from build123d import *

# Parameters (mm, degrees)
F0_R     = 3.175
F1_DEPTH = 19.05
F2_R     = 3.175
F3_DEPTH = 9.525
F4_W     = 15.875
F4_H     = 31.190733
F5_DEPTH = 9.525
F6_R     = 3.175
F7_DEPTH = 20.32
F8_R     = 3.175
F9_DEPTH = 20.32


with BuildPart() as f1:
    # F0 (on Top) → F1 (new body)
    with BuildSketch(Plane.XY):
        with BuildLine():
            ThreePointArc((100.157061, 0.559267), (119.207061, 19.609267), (100.157061, 38.659267))
            Line((100.157061, 38.659267), (-97.640359, 38.659267))
            ThreePointArc((-97.640359, 38.659267), (-116.690359, 19.609267), (-97.640359, 0.559267))
            Line((-97.640359, 0.559267), (100.157061, 0.559267))
        make_face()
        with Locations((-97.640359, 19.609267)):
            Circle(F0_R, mode=Mode.SUBTRACT)
        with Locations((100.157061, 19.609267)):
            Circle(F0_R, mode=Mode.SUBTRACT)
    extrude(amount=F1_DEPTH)

    # F2 (on face) → F3 (cut)
    with BuildSketch(Plane.XY.offset(19.05)):
        with Locations((-97.640359, 19.609267)):
            Circle(F2_R)
        with Locations((100.157061, 19.609267)):
            Circle(F2_R)
        with BuildLine():
            ThreePointArc((100.149441, -5.790733), (125.549441, 19.609267), (100.149441, 45.009267))
            Line((100.149441, 45.009267), (36.649441, 45.009267))
            Line((36.649441, 45.009267), (36.649441, -5.790733))
            Line((36.649441, -5.790733), (100.149441, -5.790733))
        make_face()
        with Locations((100.157061, 19.609267)):
            Circle(F2_R, mode=Mode.SUBTRACT)
        with BuildLine():
            Line((-34.140359, -5.790733), (-34.140359, 45.009267))
            Line((-34.140359, 45.009267), (-97.640359, 45.009267))
            ThreePointArc((-97.640359, 45.009267), (-123.040359, 19.609267), (-97.640359, -5.790733))
            Line((-97.640359, -5.790733), (-34.140359, -5.790733))
        make_face()
        with Locations((-97.640359, 19.609267)):
            Circle(F2_R, mode=Mode.SUBTRACT)
    extrude(amount=-F3_DEPTH, mode=Mode.SUBTRACT)

    # F4 (on face) → F5 (cut)
    with BuildSketch(Plane(origin=(0, 0, 0), x_dir=(1, 0, 0), z_dir=(0, 0, -1))):
        Polygon((-15.875, 0), (-15.875, -19.609267), (0, -19.609267), (15.875, -19.609267), (15.875, 0), align=None)
        with Locations((-7.9375, -35.204633)):
            Rectangle(F4_W, F4_H)
        with Locations((7.9375, -35.204633)):
            Rectangle(F4_W, F4_H)
    extrude(amount=-F5_DEPTH, mode=Mode.SUBTRACT)

    # F6 (on face) → F7 (join)
    with BuildSketch(Plane(origin=(0, 0, 0), x_dir=(1, 0, 0), z_dir=(0, 0, -1))):
        with Locations((-97.640359, -19.609267)):
            Circle(F6_R)
    extrude(amount=-F7_DEPTH)

    # F8 (on face) → F9 (join)
    with BuildSketch(Plane(origin=(0, 0, 0), x_dir=(1, 0, 0), z_dir=(0, 0, -1))):
        with Locations((100.157061, -19.609267)):
            Circle(F8_R)
    extrude(amount=-F9_DEPTH)


solid = f1.part
Work out the finished part from the listing and answer in its coordinate system (mm). A direction names the side the tool comes from. Round coordinates to 2 decimals unless told otherwise and drop trailing zeros. Write each loop counter-clockwise with the first axis right and the second up, starting at its lowest first coordinate (ties: lowest second). Pieces come first, ordered by that corner, then holes.
1) A cutting plane is placed at C-C (x = -59.5). Give the vertices of the cut face in (y, z) (3 decimals).
2) A tool of negligible diameter and unlimited length cuts with its end or side. For faces 4 (the flat face through (15.875, 20, 5)), 5 (the cylindrical face through (-116.686, 20.028, 4.696)), 6 (the cylindrical face through (-94.71, 20.83, 14.85)), from which of +Z, -Z, +X, -X, +Y, -Y can it reach the whole face along a straight path? Write none if from no direction.
3) A cutting plane is placed at D-D (y = 33). Give the vertices of the cut face in (x, z) (3 decimals), plus the area to 3 significant figures.
4) Straight lines are drawn through the part: line 1 (X direction, y = 21, z = 17.5); line 2 (Z direction, x = 53.5, y = 6) (3 decimals); line 3 (Z direction, x = -17, y = 10.5). For each, find the intervals that lie inside material, in ascending order.
5) The mould has two halves that part along X. Classify faces 1 (the flat face through (-15.875, 19, 5)), 2 (the flat face through (100, 20, 20.32)), 3 (the cylindrical face through (119.202, 19.19, 4.696)): pulls with the +X half, pulls with the -X half, needs draft (parallel to the pull), parting line crosses it, or undercut.
6) A cutting plane is placed at B-B (y = 6.5). Give the vertices of the cut face in (x, z) (3 decimals).
7) Given pin 1 Ø10.5 at (y, z) = (24.5, 15.5) entering from +X; pin 2 Ø1 at (y, z) = (17, 11) entering from +X; pin 3 Ø3 at (y, z) = (24, 14) entering from -X, each flat-ended and moving along its own axis, determine where each tip first touches the part or whether it passes through.
8) A cutting plane is placed at A-A (z = 4.75). Give the vertices of the cut face in (x, y) (3 decimals).
Completed:
1. outline: (0.559, 0) - (38.659, 0) - (38.659, 9.525) - (0.559, 9.525) - close
2. face 4: -Z, +Y, -Y
2. face 5: +Z, -Z, -X
2. face 6: +Z
3. outline: (-111.19, 0) - (-15.875, 0) - (-15.875, 9.525) - (15.875, 9.525) - (15.875, 0) - (113.707, 0) - (113.707, 9.525) - (36.649, 9.525) - (36.649, 19.05) - (-34.14, 19.05) - (-34.14, 9.525) - (-111.19, 9.525) - close
3. area: 2,510 mm2
4. line 1: x = -100.49 to -94.79, -34.14 to 36.65, 97.3 to 103.01
4. line 2: z = 0 to 9.525
4. line 3: z = 0 to 19.05
5. face 1: undercut
5. face 2: needs draft
5. face 3: pulls with the +X half
6. outline: (-111.462, 0) - (-15.875, 0) - (-15.875, 9.525) - (15.875, 9.525) - (15.875, 0) - (113.979, 0) - (113.979, 9.525) - (36.649, 9.525) - (36.649, 19.05) - (-34.14, 19.05) - (-34.14, 9.525) - (-111.462, 9.525) - close
7. pin 1: stops at x = 103.33
7. pin 2: stops at x = 102.53
7. pin 3: stops at x = -98.95
8. outline: (-97.64, 0.559) - (-15.875, 0.559) - (-15.875, 38.659) - (-97.64, 38.659) arc R19.05 ccw to start; (15.875, 0.559) - (100.157, 0.559) arc R19.05 ccw to (100.157, 38.659) - (15.875, 38.659) - close
